For this review, take the finished solid that the model builds, in its own axes (mm). Face numbers are marked on the shaded views. A direction names the side the tool comes from. Coordinates: 2 decimals unless noted, no trailing zeros. Write each loop counter-clockwise with the first axis right and the second up, starting at its lowest first coordinate (ties: lowest second). Pieces come first, ordered by that corner, then holes.
1) We need section A-A on z = 0. Write out the cut boundary in (x, y).
2) We need section B-B on x = 21.5. Write out the cut boundary in (y, z).
3) To check wall thickness, follow line 1 along X through (y, z) = (2.1, 0); line 2 along X through (y, z) = (8, 0); line 3 along Z through (x, y) = (15, 3). State the ranges of each line that lie inside material, in increasing order.
4) We need section D-D on y = 11.75. Write out the cut boundary in (x, z).
5) For the marked faces 4, 5, 6 and 7, list the 3-axis set-ups (+Z, -Z, +X, -X, +Y, -Y) from which the entire face can be reached by the end or side of a thin tool; tool diameter is ignored.
6) We need section C-C on x = 14. Write out the cut boundary in (y, z).
7) Mouldability with a two-part tool opening along X and no side actions: class the marked faces 1, 2 and 3 as pulls with the +X half, pulls with the -X half, needs draft (parallel to the pull), parting line crosses it, or undercut.
8) Insertion check: P1, Ø1.5, axis at x = -7, y = 4, coming from the +Z side; P2, Ø3, axis at x = 20.64, z = 0, coming from the +Y side; P3, Ø4, axis at y = 5.5, z = -7, coming from the +X side; P4, Ø4.5, axis at x = 10, y = 2, coming from the -Z side. Each pin has a flat end and moves straight along its axis. Give the tip position at first contact, or say it passes through.
from build123d import *

# Parameters (mm, degrees)
SKETCH1_R           = 1.75
BOSS_EXTRUDE1_DEPTH = 4
SKETCH_1_R          = 3.65
CUT_EXTRUDE_1_DEPTH = 29.890195164
SKETCH_2_R          = 5.65
SKETCH_2_R_2        = 3.65
EXTRUDE_1_DEPTH     = 10


with BuildPart() as part:
    # Sketch1 → Boss-Extrude1 (new body)
    with BuildSketch(Plane(origin=(0, 4, 0), x_dir=(1, 0, 0), z_dir=(0, 1, 0))):
        with BuildLine():
            Line((1.305695063, -4), (20.643657446, -4))
            ThreePointArc((20.643657446, -4), (24.643657446, 0), (20.643657446, 4))
            Line((20.643657446, 4), (2.081641936, 4))
            ThreePointArc((2.081641936, 4), (2.861028333, 4.588201733), (3.521749436, 5.30713988))
            ThreePointArc((3.521749436, 5.30713988), (3.405395609, 5.596745198), (3.282888305, 5.883801663))
            ThreePointArc((3.282888305, 5.883801663), (1.93527598, 5.894040025), (0.627094961, 5.57027124))
            ThreePointArc((0.627094961, 5.57027124), (0.366286148, 6.046375), (0.084372603, 6.510293938))
            ThreePointArc((0.084372603, 6.510293938), (1.018855105, 7.48132754), (1.683794586, 8.65351323))
            ThreePointArc((1.683794586, 8.65351323), (1.496450048, 8.903135899), (1.303821399, 9.148703928))
            ThreePointArc((1.303821399, 9.148703928), (-0.000522033, 8.809805691), (-1.180330337, 8.158486898))
            ThreePointArc((-1.180330337, 8.158486898), (-1.555477026, 8.550865528), (-1.947855656, 8.926012217))
            ThreePointArc((-1.947855656, 8.926012217), (-1.296536862, 10.105820521), (-0.957638625, 11.410163953))
            ThreePointArc((-0.957638625, 11.410163953), (-1.203206655, 11.602792602), (-1.452829324, 11.79013714))
            ThreePointArc((-1.452829324, 11.79013714), (-2.625015014, 11.125197659), (-3.596048616, 10.190715157))
            ThreePointArc((-3.596048616, 10.190715157), (-4.059967554, 10.472628702), (-4.536071314, 10.733437515))
            ThreePointArc((-4.536071314, 10.733437515), (-4.212302529, 12.041618533), (-4.222540891, 13.389230859))
            ThreePointArc((-4.222540891, 13.389230859), (-4.509597355, 13.511738163), (-4.799202674, 13.62809199))
            ThreePointArc((-4.799202674, 13.62809199), (-5.759348103, 12.682425791), (-6.455432668, 11.528463019))
            ThreePointArc((-6.455432668, 11.528463019), (-6.976508546, 11.680699536), (-7.503891752, 11.809396783))
            ThreePointArc((-7.503891752, 11.809396783), (-7.529737283, 13.156800143), (-7.888414517, 14.455843809))
            ThreePointArc((-7.888414517, 14.455843809), (-8.197396993, 14.499881098), (-8.507248835, 14.537314892))
            ThreePointArc((-8.507248835, 14.537314892), (-9.18992168, 13.375367565), (-9.563620196, 12.080565177))
            ThreePointArc((-9.563620196, 12.080565177), (-10.106342554, 12.09275), (-10.649064912, 12.080565177))
            ThreePointArc((-10.649064912, 12.080565177), (-11.022763428, 13.375367565), (-11.705436272, 14.537314892))
            ThreePointArc((-11.705436272, 14.537314892), (-12.015288115, 14.499881098), (-12.324270591, 14.455843809))
            ThreePointArc((-12.324270591, 14.455843809), (-12.682947825, 13.156800143), (-12.708793355, 11.809396783))
            ThreePointArc((-12.708793355, 11.809396783), (-13.236176561, 11.680699536), (-13.757252439, 11.528463019))
            ThreePointArc((-13.757252439, 11.528463019), (-14.453337005, 12.682425791), (-15.413482434, 13.62809199))
            ThreePointArc((-15.413482434, 13.62809199), (-15.703087752, 13.511738163), (-15.990144217, 13.389230859))
            ThreePointArc((-15.990144217, 13.389230859), (-16.000382579, 12.041618533), (-15.676613793, 10.733437515))
            ThreePointArc((-15.676613793, 10.733437515), (-16.152717554, 10.472628702), (-16.616636492, 10.190715157))
            ThreePointArc((-16.616636492, 10.190715157), (-17.587670094, 11.125197659), (-18.759855783, 11.79013714))
            ThreePointArc((-18.759855783, 11.79013714), (-19.009478453, 11.602792602), (-19.255046482, 11.410163953))
            ThreePointArc((-19.255046482, 11.410163953), (-18.916148245, 10.105820521), (-18.264829452, 8.926012217))
            ThreePointArc((-18.264829452, 8.926012217), (-18.657208082, 8.550865528), (-19.032354771, 8.158486898))
            ThreePointArc((-19.032354771, 8.158486898), (-20.212163074, 8.809805691), (-21.516506507, 9.148703928))
            ThreePointArc((-21.516506507, 9.148703928), (-21.709135156, 8.903135899), (-21.896479694, 8.65351323))
            ThreePointArc((-21.896479694, 8.65351323), (-21.231540213, 7.48132754), (-20.297057711, 6.510293938))
            ThreePointArc((-20.297057711, 6.510293938), (-20.578971255, 6.046375), (-20.839780068, 5.57027124))
            ThreePointArc((-20.839780068, 5.57027124), (-22.147961087, 5.894040025), (-23.495573413, 5.883801663))
            ThreePointArc((-23.495573413, 5.883801663), (-23.618080717, 5.596745198), (-23.734434544, 5.30713988))
            ThreePointArc((-23.734434544, 5.30713988), (-22.788768345, 4.346994451), (-21.634805572, 3.650909885))
            ThreePointArc((-21.634805572, 3.650909885), (-21.78704209, 3.129834008), (-21.915739337, 2.602450802))
            ThreePointArc((-21.915739337, 2.602450802), (-23.263142697, 2.576605271), (-24.562186363, 2.217928037))
            ThreePointArc((-24.562186363, 2.217928037), (-24.606223651, 1.908945561), (-24.643657446, 1.599093719))
            ThreePointArc((-24.643657446, 1.599093719), (-23.481710119, 0.916420874), (-22.186907731, 0.542722358))
            ThreePointArc((-22.186907731, 0.542722358), (-12.402167869, -11.872817218), (1.305695063, -4))
        make_face()
        with Locations(Location((20.643657446, 0, 0), (0, 0, 90))):
            Circle(SKETCH1_R, mode=Mode.SUBTRACT)
    extrude(amount=-BOSS_EXTRUDE1_DEPTH)

    # 草图1 → 切除-拉伸1 (cut, through all)
    with BuildSketch(Plane.XZ):
        with Locations(Location((-10.106342554, 0, 0), (0, 0, 270))):
            Circle(SKETCH_1_R)
    extrude(amount=-CUT_EXTRUDE_1_DEPTH, mode=Mode.SUBTRACT)

    # 草图2 → 凸台-拉伸1 (add)
    with BuildSketch(Plane(origin=(0, 4, 0), x_dir=(1, 0, 0), z_dir=(0, 1, 0))):
        with Locations(Location((-10.106342554, 0, 0), (0, 0, 270))):
            Circle(SKETCH_2_R)
        with Locations(Location((-10.106342554, 0, 0), (0, 0, 90))):
            Circle(SKETCH_2_R_2, mode=Mode.SUBTRACT)
    extrude(amount=EXTRUDE_1_DEPTH)


solid = part.part
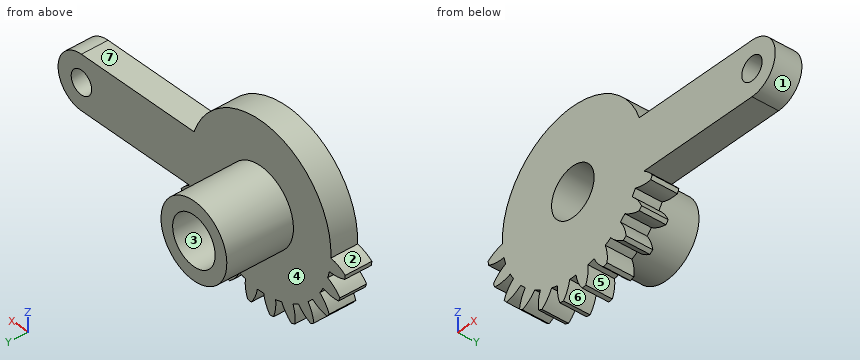
Result:
1. outline: (-22.2, 0) - (-13.76, 0) - (-13.76, 14) - (-15.76, 14) - (-15.76, 4) - (-22.2, 4) - close; (-6.46, 0) - (18.89, 0) - (18.89, 4) - (-4.46, 4) - (-4.46, 14) - (-6.46, 14) - close; (22.39, 0) - (24.64, 0) - (24.64, 4) - (22.39, 4) - close
2. outline: (0, -3.91) - (4, -3.91) - (4, -1.53) - (0, -1.53) - close; (0, 1.53) - (4, 1.53) - (4, 3.91) - (0, 3.91) - close
3. line 1: x = -22.2 to -13.76, -6.46 to 18.89, 22.39 to 24.64
3. line 2: x = -15.76 to -13.76, -6.46 to -4.46
3. line 3: z = -4 to 4
4. outline: circle Ø11.3 at (-10.11, 0); hole circle Ø7.3 at (-10.11, 0)
5. face 4: +Y
5. face 5: +Y, -Y
5. face 6: -Z, +Y, -Y
5. face 7: +Z, +X, +Y, -Y
6. outline: (0, -4) - (4, -4) - (4, 4) - (0, 4) - close
7. face 1: pulls with the +X half
7. face 2: pulls with the -X half
7. face 3: undercut
8. P1: stops at z = 11.86
8. P2: passes through
8. P3: stops at x = 3.37
8. P4: stops at z = -4
